from build123d import *

# Parameters (mm, degrees)
F2_DEPTH = 11
F3_R     = 6.25
F4_DEPTH = 5.001
F5_R     = 5
F6_R     = 8.6
F7_DEPTH = 1


# Not quite as in the source:
# - a pattern or mirror of a feature is missing from the dataset's text; its kind, count and spacing are read off the source's solid


with BuildPart() as f2:
    # F1 (on Front) → F2 (new body, symmetric)
    with BuildSketch(Plane.XZ):
        with BuildLine():
            ThreePointArc((9.0862533533, 5), (0, 0.2), (-9.0862533533, 5))
            Line((-9.0862533533, 5), (-10.95, 5))
            Line((-10.95, 5), (-10.95, 0))
            Line((-10.95, 0), (-29, 0))
            Line((-29, 0), (-29, -5))
            Line((-29, -5), (29, -5))
            Line((29, -5), (29, 0))
            Line((29, 0), (10.95, 0))
            Line((10.95, 0), (10.95, 5))
            Line((10.95, 5), (9.0862533533, 5))
        make_face()
    extrude(amount=F2_DEPTH, both=True)

    # F3 (on Top) → F4 (cut, through all)
    with BuildSketch(Plane.XY):
        with Locations((-19, 0)):
            Circle(F3_R)
    f4 = extrude(amount=-F4_DEPTH, mode=Mode.SUBTRACT)

    # F4_copies: F4 across plane
    add(f4.mirror(Plane(origin=(0, 0, 0), x_dir=(0, 0, 1), z_dir=(1, 0, 0))), mode=Mode.SUBTRACT)

    # F5
    f5_edges = [f2.edges().sort_by_distance(p)[0] for p in [
        (-29, -11, -2.5),
        (-29, 11, -2.5),
        (29, -11, -2.5),
        (29, 11, -2.5),
    ]]
    fillet(f5_edges, radius=F5_R)

    # F6 (on face) → F7 (cut)
    with BuildSketch(Plane(origin=(0, 0, -5), x_dir=(1, 0, 0), z_dir=(0, 0, -1))):
        with Locations((-19, 0)):
            Circle(F6_R)
        with Locations((19, 0)):
            Circle(F6_R)
    extrude(amount=-F7_DEPTH, mode=Mode.SUBTRACT)


solid = f2.part
Work out the finished part from the listing and answer in its coordinate system (mm). A direction names the side the tool comes from. Coordinates: 2 decimals unless noted, no trailing zeros. Write each loop counter-clockwise with the first axis right and the second up, starting at its lowest first coordinate (ties: lowest second). Pieces come first, ordered by that corner, then holes.
1. The part is cut by section C-C, the plane z = -2.25. Write down the section's boundary in (x, y).
Results list:
outline: (-29, -6) arc R5 ccw to (-24, -11) - (24, -11) arc R5 ccw to (29, -6) - (29, 6) arc R5 ccw to (24, 11) - (-24, 11) arc R5 ccw to (-29, 6) - close; hole circle Ø12.5 at (-19, 0); hole circle Ø12.5 at (19, 0)
2. The part is cut by section D-D, the plane y = -2.5. Write down the section's boundary in (x, z).
Results list:
outline: (-29, -5) - (-27.23, -5) - (-27.23, -4) - (-24.73, -4) - (-24.73, 0) - (-29, 0) - close; (-13.27, -4) - (-10.77, -4) - (-10.77, -5) - (10.77, -5) - (10.77, -4) - (13.27, -4) - (13.27, 0) - (10.95, 0) - (10.95, 5) - (9.09, 5) arc R11 cw to (-9.09, 5) - (-10.95, 5) - (-10.95, 0) - (-13.27, 0) - close; (24.73, -4) - (27.23, -4) - (27.23, -5) - (29, -5) - (29, 0) - (24.73, 0) - close
3. The part is cut by section A-A, the plane y = 0. Write down the section's boundary in (x, z).
Results list:
outline: (-29, -5) - (-27.6, -5) - (-27.6, -4) - (-25.25, -4) - (-25.25, 0) - (-29, 0) - close; (-12.75, -4) - (-10.4, -4) - (-10.4, -5) - (10.4, -5) - (10.4, -4) - (12.75, -4) - (12.75, 0) - (10.95, 0) - (10.95, 5) - (9.09, 5) arc R11 cw to (-9.09, 5) - (-10.95, 5) - (-10.95, 0) - (-12.75, 0) - close; (25.25, -4) - (27.6, -4) - (27.6, -5) - (29, -5) - (29, 0) - (25.25, 0) - close
4. The part is cut by section B-B, the plane x = 19. Write down the section's boundary in (y, z), and give its area (3 significant figures).
Results list:
outline: (-11, -5) - (-8.6, -5) - (-8.6, -4) - (-6.25, -4) - (-6.25, 0) - (-11, 0) - close; (6.25, -4) - (8.6, -4) - (8.6, -5) - (11, -5) - (11, 0) - (6.25, 0) - close
area: 42.8 mm2
5. Consider line 1 along X through (y, z) = (0, -4.75); line 2 along Y through (x, z) = (-19, -4.6); line 3 along Y through (x, z) = (19, -2.4). Determine where each line is inside the solid, lowest interval first.
Results list:
line 1: x = -29 to -27.6, -10.4 to 10.4, 27.6 to 29
line 2: y = -11 to -8.6, 8.6 to 11
line 3: y = -11 to -6.25, 6.25 to 11
6. For faces 1 (the cylindrical face through (-11.056, 3.294, -4.507)), 2 (the flat face through (-10.95, 0, 3)), 3 (the flat face through (26, 0, 0)), determine the directions among +Z, -Z, +X, -X, +Y, -Y from which every point of the face is accessible in a straight line to the end or side of a thin tool.
Results list:
face 1: -Z
face 2: +Z, -X, +Y, -Y
face 3: +Z, +X, +Y, -Y
7. Flat-ended cylindrical pins translate along their axes: pin 1 (5.5 mm diameter, centred on y = -1, z = 3.5, fed in from -X); pin 2 (2 mm diameter, centred on y = 0.5, z = 4, fed in from +X); pin 3 (1.5 mm diameter, centred on x = -17.5, z = 2.5, fed in from +Y); pin 4 (9 mm diameter, centred on x = -21, y = 5, fed in from +Z). Find the tip coordinate at first contact, or state that the pin passes through.
Results list:
pin 1: stops at x = -10.95
pin 2: stops at x = 10.95
pin 3: passes through
pin 4: stops at z = 0
